```python
from build123d import *

# Parameters (mm, degrees)
SKETCH_1_R          = 2.1
SKETCH_1_R_2        = 41.1
EXTRUDE_1_DEPTH     = 3
SKETCH_2_R          = 2.1
CUT_EXTRUDE_1_DEPTH = 3


with BuildPart() as part:
    # 草图1 → 凸台-拉伸1 (new body)
    with BuildSketch(Plane.XY):
        with BuildLine():
            Line((0, 49), (115, 49))
            ThreePointArc((115, 49), (118.535533906, 47.535533906), (120, 44))
            Line((120, 44), (120, 24))
            ThreePointArc((120, 24), (118.535533906, 20.464466094), (115, 19))
            Line((115, 19), (79, 19))
            ThreePointArc((79, 19), (77.086582838, 18.619397663), (75.464466094, 17.535533906))
            Line((75.464466094, 17.535533906), (61.464466094, 3.535533906))
            ThreePointArc((61.464466094, 3.535533906), (60, 0), (61.464466094, -3.535533906))
            Line((61.464466094, -3.535533906), (75.464466094, -17.535533906))
            ThreePointArc((75.464466094, -17.535533906), (77.086582838, -18.619397663), (79, -19))
            Line((79, -19), (115, -19))
            ThreePointArc((115, -19), (118.535533906, -20.464466094), (120, -24))
            Line((120, -24), (120, -44))
            ThreePointArc((120, -44), (118.535533906, -47.535533906), (115, -49))
            Line((115, -49), (0, -49))
            ThreePointArc((0, -49), (-49, 0), (0, 49))
        make_face()
        with Locations((-45, 0)):
            Circle(SKETCH_1_R, mode=Mode.SUBTRACT)
        with Locations((-22.5, 38.97114317)):
            Circle(SKETCH_1_R, mode=Mode.SUBTRACT)
        with Locations((22.5, 38.97114317)):
            Circle(SKETCH_1_R, mode=Mode.SUBTRACT)
        with Locations((45, 0)):
            Circle(SKETCH_1_R, mode=Mode.SUBTRACT)
        with Locations((22.5, -38.97114317)):
            Circle(SKETCH_1_R, mode=Mode.SUBTRACT)
        with Locations((-22.5, -38.97114317)):
            Circle(SKETCH_1_R, mode=Mode.SUBTRACT)
        Circle(SKETCH_1_R_2, mode=Mode.SUBTRACT)
        with BuildLine():
            Line((93, -42), (107, -42))
            ThreePointArc((107, -42), (109.121320344, -41.121320344), (110, -39))
            Line((110, -39), (110, -29))
            ThreePointArc((110, -29), (109.121320344, -26.878679656), (107, -26))
            Line((107, -26), (93, -26))
            ThreePointArc((93, -26), (90.878679656, -26.878679656), (90, -29))
            Line((90, -29), (90, -39))
            ThreePointArc((90, -39), (90.878679656, -41.121320344), (93, -42))
        make_face(mode=Mode.SUBTRACT)
        with BuildLine():
            Line((34.394767044, -42), (76, -42))
            ThreePointArc((76, -42), (78.121320344, -41.121320344), (79, -39))
            Line((79, -39), (79, -32.213203436))
            ThreePointArc((79, -32.213203436), (78.771638598, -31.065153138), (78.121320344, -30.091883092))
            Line((78.121320344, -30.091883092), (54.908116908, -6.878679656))
            ThreePointArc((54.908116908, -6.878679656), (53.934846861, -6.228361402), (52.786796564, -6))
            Line((52.786796564, -6), (51.215232109, -6))
            ThreePointArc((51.215232109, -6), (49.28620286, -6.702426029), (48.26050718, -8.480769231))
            ThreePointArc((48.26050718, -8.480769231), (42.740359483, -23.963757452), (32.410453561, -36.75))
            ThreePointArc((32.410453561, -36.75), (31.588524004, -40.060660172), (34.394767044, -42))
        make_face(mode=Mode.SUBTRACT)
        with BuildLine():
            Line((93, 26), (107, 26))
            ThreePointArc((107, 26), (109.121320344, 26.878679656), (110, 29))
            Line((110, 29), (110, 39))
            ThreePointArc((110, 39), (109.121320344, 41.121320344), (107, 42))
            Line((107, 42), (93, 42))
            ThreePointArc((93, 42), (90.878679656, 41.121320344), (90, 39))
            Line((90, 39), (90, 29))
            ThreePointArc((90, 29), (90.878679656, 26.878679656), (93, 26))
        make_face(mode=Mode.SUBTRACT)
        with BuildLine():
            Line((51.215232109, 6), (52.786796564, 6))
            ThreePointArc((52.786796564, 6), (53.934846861, 6.228361402), (54.908116908, 6.878679656))
            Line((54.908116908, 6.878679656), (78.121320344, 30.091883092))
            ThreePointArc((78.121320344, 30.091883092), (78.771638598, 31.065153139), (79, 32.213203436))
            Line((79, 32.213203436), (79, 39))
            ThreePointArc((79, 39), (78.121320344, 41.121320344), (76, 42))
            Line((76, 42), (34.394767044, 42))
            ThreePointArc((34.394767044, 42), (31.588524004, 40.060660172), (32.410453561, 36.75))
            ThreePointArc((32.410453561, 36.75), (42.740359483, 23.963757452), (48.26050718, 8.480769231))
            ThreePointArc((48.26050718, 8.480769231), (49.28620286, 6.702426029), (51.215232109, 6))
        make_face(mode=Mode.SUBTRACT)
    extrude(amount=EXTRUDE_1_DEPTH)

    # 草图2 → 切除-拉伸1 (cut)
    with BuildSketch(Plane.XY):
        with Locations((85, 44)):
            Circle(SKETCH_2_R)
        with Locations((115, 44)):
            Circle(SKETCH_2_R)
        with Locations(Location((115, 24, 0), (0, 0, 180))):
            Circle(SKETCH_2_R)
        with Locations(Location((85, 24, 0), (0, 0, 180))):
            Circle(SKETCH_2_R)
        with Locations((85, -24)):
            Circle(SKETCH_2_R)
        with Locations((115, -24)):
            Circle(SKETCH_2_R)
        with Locations(Location((115, -44, 0), (0, 0, 180))):
            Circle(SKETCH_2_R)
        with Locations(Location((85, -44, 0), (0, 0, 180))):
            Circle(SKETCH_2_R)
    extrude(amount=CUT_EXTRUDE_1_DEPTH, mode=Mode.SUBTRACT)


solid = part.part
```
CAD build for the part. Positions are in the model's coordinates, mm. A direction names the side the tool comes from. Round coordinates to 2 decimals unless told otherwise and drop trailing zeros. Loops run counter-clockwise (first coordinate to the right, second up) from the corner with the lowest first, then second, coordinate; pieces in that order, holes last. Notation, with made-up numbers: (19.25, 34.25) - (77.25, 34.25) arc R15 cw to (77.25, 45.25) - close; hole circle Ø2 at (11, 16.25). An arc over 180 degrees is marked (long way). Return JSON: item names as keys, results as strings. Group by question number.
Q1. Tool access for faces 1 (the face through (66.68, -18.65, 1.48)), 2 (the face through (119, 21, 1)): list every direction of +Z, -Z, +X, -X, +Y, -Y with a clear straight run to the whole face (end or side of a thin tool).
Q2. Band-saw the part on D-D on x = -45. Give the cut face in (y, z).
Q3. Band-saw the part on A-A on y = 0. Give the cut face in (x, z).
Q4. Band-saw the part on C-C on x = 36. Give the cut face in (y, z), plus the area to 3 significant figures.
Q5. Band-saw the part on B-B on x = 81. Give the cut face in (y, z), plus the area to 3 significant figures.
Q6. Flat gauge pins, fed straight in: pin 1 Ø1.5 at (x, z) = (-1.5, 1.5) entering from +Y; pin 2 Ø1 at (x, y) = (37.5, 34.5) entering from +Z; pin 3 Ø1.5 at (y, z) = (-35.5, 1) entering from -X; pin 4 Ø0.9 at (y, z) = (-37, 2) entering from -X. Where does each tip first touch, or does it go through?
Q7. Drill centre lines: line 1 along Y through (x, z) = (85, 1.45); line 2 along Y through (x, z) = (70.5, 2.45); line 3 along X through (y, z) = (27, 2.3). Where is each one in solid material? Low to high. Write a range as [from, to].
Q8. Two-plate mould, pull along Y, no slides. Class faces 3 (the face through (90, -34, 1)), 4 (the face through (-48.99, -1.08, 1.48)), 5 (the face through (120, 34, 1)): +Y half, -Y half, draft (parallel to the pull), parting line (faces both ways), or undercut.
Solutions:
{
 "1": {"face 1": "+Z, -Z", "face 2": "+Z, -Z, +X"},
 "2": {"outline": "(-19.39, 0) - (-2.1, 0) - (-2.1, 3) - (-19.39, 3) - close; (2.1, 0) - (19.39, 0) - (19.39, 3) - (2.1, 3) - close"},
 "3": {"outline": "(-49, 0) - (-47.1, 0) - (-47.1, 3) - (-49, 3) - close; (-42.9, 0) - (-41.1, 0) - (-41.1, 3) - (-42.9, 3) - close; (41.1, 0) - (42.9, 0) - (42.9, 3) - (41.1, 3) - close; (47.1, 0) - (60, 0) - (60, 3) - (47.1, 3) - close"},
 "4": {"outline": "(-49, 0) - (-42, 0) - (-42, 3) - (-49, 3) - close; (-33.24, 0) - (-19.83, 0) - (-19.83, 3) - (-33.24, 3) - close; (19.83, 0) - (33.24, 0) - (33.24, 3) - (19.83, 3) - close; (42, 0) - (49, 0) - (49, 3) - (42, 3) - close", "area": "122 mm^2"},
 "5": {"outline": "(-49, 0) - (-19, 0) - (-19, 3) - (-49, 3) - close; (19, 0) - (49, 0) - (49, 3) - (19, 3) - close", "area": "180 mm^2"},
 "6": {"pin 1": "stops at y = 48.99", "pin 2": "passes through", "pin 3": "stops at x = -34.55", "pin 4": "stops at x = -32.64"},
 "7": {"line 1": "y = [-49, -46.1], [-41.9, -26.1], [-21.9, -19], [19, 21.9], [26.1, 41.9], [46.1, 49]", "line 2": "y = [-49, -42], [-22.47, -12.57], [12.57, 22.47], [42, 49]", "line 3": "x = [-40.89, -30.99], [30.99, 40.89], [75.03, 90.76], [109.24, 120]"},
 "8": {"face 3": "undercut", "face 4": "parting line", "face 5": "draft"}
}
